Autodesk Inventor part; units mm, degrees
ref_plane "Work Plane1" through (0, 0, 61.5) normal (0, 0, 1) x (1, 0, 0)
ref_plane "Work Plane2" through (0, 61.5, 0) normal (0, 1, 0) x (-1, 0, 0)
ref_plane "Work Plane3" through (26.75, 0, 0) normal (1, 0, 0) x (0, 1, 0)
ref_plane "Work Plane1" through (0, 0, 61.5) normal (0, 0, 1) x (1, 0, 0)
sketch "Sketch1" plane through (0, 0, 61.5) normal (0, 0, 1) x (1, 0, 0)
  circle A0 centre (0, 0) radius 13.25
  dimension "d1" = 26.5
ref_plane "Work Plane2" through (0, 61.5, 0) normal (0, 1, 0) x (-1, 0, 0)
sketch "Sketch2" plane through (0, 61.5, 0) normal (0, 1, 0) x (-1, 0, 0)
  circle A0 centre (0, 0) radius 13.25
  dimension "d3" = 26.5
sketch "Sketch3" plane through (0, 0, 0) normal (1, 0, 0) x (0, 1, 0)
  line L0 (13.25, 61.5) -> (-13.25, 61.5) construction
  line L1 (61.5, -13.25) -> (61.5, 13.25) construction
  line L2 (0, -28.2) -> (0, 76.45) construction
  line L3 (-28.2, 0) -> (76.45, 0) construction
  line L4 (0, 0) -> (0, 61.5)
  line L5 (0, 0) -> (61.5, 0)
  line L6 (61.5, 13.25) -> (28.25, 13.25)
  line L7 (13.25, 28.25) -> (13.25, 61.5)
  arc A0 (13.25, 28.25) -> (28.25, 13.25) centre (28.25, 28.25) ccw
  dimension "d4" = 15
sweep "Sweep1" add profiles "Sketch1" path "Sketch3" path curves L7 A0 L6
shell "Shell1" thickness 0.5 removed faces 2 at (0.1548, 61.5, -7.494) at (-0.404, -5.4414, 61.5)
ref_plane "Work Plane3" through (26.75, 0, 0) normal (1, 0, 0) x (0, 1, 0)
sketch "Sketch4" plane through (26.75, 0, 0) normal (1, 0, 0) x (0, 1, 0)
  circle A0 centre (8.6449, 8.6449) radius 2.5
  point P0 (0, 0)
extrude "Extrusion1" cut sketch "Sketch4" against normal through all
properties part number "knee 90"
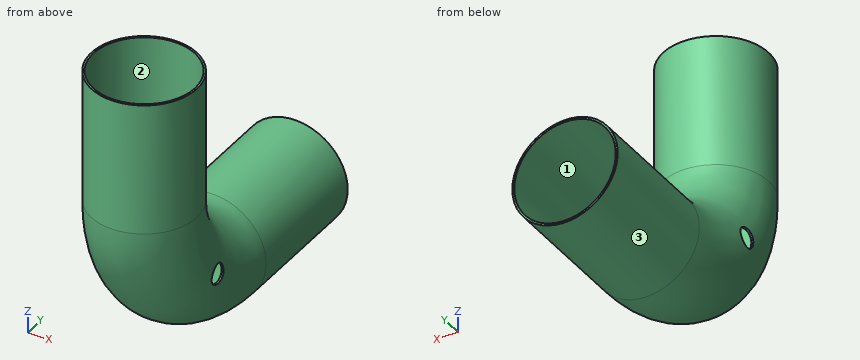
Here's how the part is built. I have some questions about the finished solid (model axes, mm). Face numbers are marked on the shaded views. Round coordinates to 2 decimals unless told otherwise and drop trailing zeros. Loops run counter-clockwise (first coordinate to the right, second up) from the corner with the lowest first, then second, coordinate; pieces in that order, holes last.
1. Suppose I cut it at D-D, the plane x = 7. Please give me the cut outline in (y, z).
Answers:
outline: (-11.25, 28.25) arc R39.5 ccw to (28.25, -11.25) - (61.5, -11.25) - (61.5, -10.66) - (28.25, -10.66) arc R38.91 cw to (-10.66, 28.25) - (-10.66, 61.5) - (-11.25, 61.5) - close; (10.66, 28.25) arc R17.59 ccw to (28.25, 10.66) - (61.5, 10.66) - (61.5, 11.25) - (28.25, 11.25) arc R17 cw to (11.25, 28.25) - (11.25, 61.5) - (10.66, 61.5) - close
2. Will these pins go through, and if not, where does the flat tip stop? pin 1 (8 mm diameter, centred on x = -10, z = 30, fed in from -Y); pin 2 (1.5 mm diameter, centred on x = -1, z = 4, fed in from +Y); pin 3 (4 mm diameter, centred on y = 8.64, z = 8.64, fed in from +X); pin 4 (10 mm diameter, centred on y = 17, z = 35.5, fed in from -X).
Answers:
pin 1: stops at y = -11.81
pin 2: stops at y = -4.19
pin 3: passes through
pin 4: stops at x = -5.62
3. Thinking about a two-plate mould opening in Z: for the marked faces 1, 2 and 3, which applies, released by +Z, released by -Z, zero draft, split by the parting line, or undercut?
Answers:
face 1: undercut
face 2: zero draft
face 3: split by the parting line
4. Suppose I cut it at A-A, the plane x = 0. Please give me the cut outline in (y, z).
Answers:
outline: (-13.25, 28.25) arc R41.5 ccw to (28.25, -13.25) - (61.5, -13.25) - (61.5, -12.75) - (28.25, -12.75) arc R41 cw to (-12.75, 28.25) - (-12.75, 61.5) - (-13.25, 61.5) - close; (12.75, 28.25) arc R15.5 ccw to (28.25, 12.75) - (61.5, 12.75) - (61.5, 13.25) - (28.25, 13.25) arc R15 cw to (13.25, 28.25) - (13.25, 61.5) - (12.75, 61.5) - close
5. Suppose I cut it at B-B, the plane y = 31.5. Please give me the cut outline in (x, z).
Answers:
outline: circle Ø26.5 at (0, 0); hole circle Ø25.5 at (0, 0)
6. If I drill on probe 1 along Z at (x, y) = (0, 41); probe 2 along X at (y, z) = (47, -0.5); probe 3 along Y at (x, z) = (2.5, 42), over which ranges is the centre line in solid material (lowest first)?
Answers:
probe 1: z = -13.25 to -12.75, 12.75 to 13.25
probe 2: x = -13.24 to -12.74, 12.74 to 13.24
probe 3: y = -13.01 to -12.5, 12.5 to 13.01
